Work out the finished part from the listing and answer in its coordinate system (mm). Face numbers are marked on the shaded views. A direction names the side the tool comes from. Give positions to 0.01 mm unless a question says otherwise; leave off trailing zeros. Loops run counter-clockwise (first coordinate to the right, second up) from the corner with the lowest first, then second, coordinate; pieces in that order, holes last. Notation, with made-up numbers: M 37,39.5 L 77,39.5 A20 cw 77,61.5 Z; hole C -27.5,22.25 d10. An arc over 180 degrees is marked long. Write item = value, one per line. Start each with the question number.
1. Flat-ended cylindrical pins translate along their axes: pin 1 Ø1.5 at (y, z) = (-14, 14) entering from -X; pin 2 Ø1 at (x, y) = (-30, -9) entering from +Z; pin 3 Ø0.5 at (y, z) = (20, -1.5) entering from -X; pin 4 Ø25 at (x, y) = (0, 0) entering from +Z. Find the tip coordinate at first contact, or state that the pin passes through.
2. The mould has two halves that part along X. Classify the marked faces 5, 6, 7 and 8: released by +X, released by -X, zero draft, split by the parting line, or undercut.
3. For the marked faces 1, 2, 3 and 4, determine the directions among +Z, -Z, +X, -X, +Y, -Y from which every point of the face is accessible in a straight line to the end or side of a thin tool.
4. Section B-B on x = 0 is taken. Determine the outline of the cut face in (y, z).
5. Section A-A on z = 13.25 is taken. Determine the outline of the cut face in (x, y).
6. Section C-C on y = 13 is taken. Determine the outline of the cut face in (x, z), plus the area to 3 significant figures.
7. Consider L1, parallel to X at y = -7, z = 5.5; L2, parallel to Y at x = 56, z = 21.85; L3, parallel to Z at x = 11.5, y = 19. Determine where each line is inside the solid, lowest interval first. Write a range as [from, to].
8. Section D-D on y = 0 is taken. Give the number of separate pieces and of enclosed holes in the cut face, plus the area to 3 significant figures.
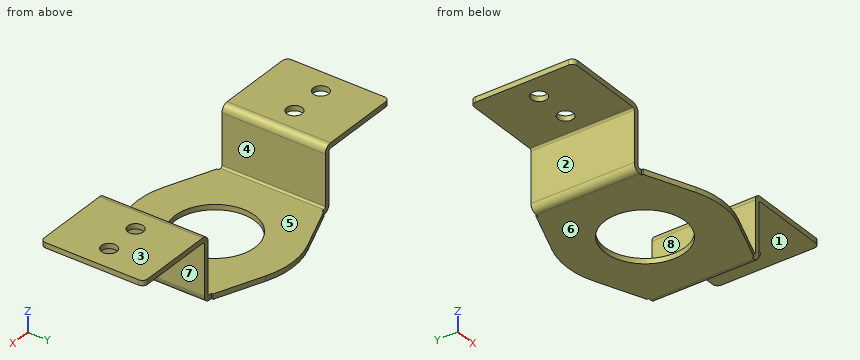
```python
from build123d import *

# Parameters (mm, degrees)
SKETCH1_R                       = 15.5
BASE_FLANGE1_DEPTH              = 2
EDGE_FLANGE1_STRIP_W            = 9.4732
EDGE_FLANGE1_STRIP_H            = 2
EDGE_FLANGE1_STRIP_CUT_DEPTH    = 40
EDGE_FLANGE1_RELIEF_W           = 10.4732
EDGE_FLANGE1_RELIEF_H           = 1
EDGE_FLANGE1_RELIEF_CUT_DEPTH   = 2
EDGE_FLANGE1_STRIP_2_W          = 9.4732
EDGE_FLANGE1_STRIP_2_H          = 2
EDGE_FLANGE1_STRIP_CUT_2_DEPTH  = 40
EDGE_FLANGE1_RELIEF_2_W         = 10.4732
EDGE_FLANGE1_RELIEF_2_H         = 1
EDGE_FLANGE1_RELIEF_CUT_2_DEPTH = 2
EDGE_FLANGE1_DEPTH              = 40
EDGE_FLANGE1_BEND_DEPTH         = 40
EDGE_FLANGE2_STRIP_W            = 9.4732
EDGE_FLANGE2_STRIP_H            = 2
EDGE_FLANGE2_STRIP_CUT_DEPTH    = 40
EDGE_FLANGE2_STRIP_2_W          = 9.4732
EDGE_FLANGE2_STRIP_2_H          = 2
EDGE_FLANGE2_STRIP_CUT_2_DEPTH  = 40
EDGE_FLANGE2_DEPTH              = 40
EDGE_FLANGE2_BEND_DEPTH         = 40
SKETCH17_R                      = 3
CUT_EXTRUDE1_DEPTH              = 10
FILLET1_R                       = 2


# Sheet-metal steps are written as plain solids
with BuildPart() as part:
    # Sketch1 → Base-Flange1 (new body)
    with BuildSketch(Plane.XY):
        with BuildLine():
            Line((-31, 20), (-11.034132012, 27.897095382))
            ThreePointArc((-11.034132012, 27.897095382), (0, 30), (11.034132012, 27.897095382))
            Line((11.034132012, 27.897095382), (31, 20))
            Line((31, 20), (31, -20))
            Line((31, -20), (11.034132012, -27.897095382))
            ThreePointArc((11.034132012, -27.897095382), (0, -30), (-11.034132012, -27.897095382))
            Line((-11.034132012, -27.897095382), (-31, -20))
            Line((-31, -20), (-31, 20))
        make_face()
        Circle(SKETCH1_R, mode=Mode.SUBTRACT)
    extrude(amount=-BASE_FLANGE1_DEPTH)

    # Edge-Flange1 strip (across the edge) → Edge-Flange1 strip cut (cut)
    with BuildSketch(Plane(origin=(-31, 20, 0), x_dir=(1, 0, 0), z_dir=(0, -1, 0))):
        with Locations((-4, -1)):
            Rectangle(EDGE_FLANGE1_STRIP_W, EDGE_FLANGE1_STRIP_H)
    extrude(amount=EDGE_FLANGE1_STRIP_CUT_DEPTH, mode=Mode.SUBTRACT)

    # Edge-Flange1 relief (on the sheet) → Edge-Flange1 relief cut (cut)
    with BuildSketch(Plane(origin=(-30.2634, 20, 0), x_dir=(1, 0, 0), z_dir=(0, 0, 1))):
        with Locations((-4.2366, 0.5)):
            Rectangle(EDGE_FLANGE1_RELIEF_W, EDGE_FLANGE1_RELIEF_H)
        with Locations((-4.2366, -40.5)):
            Rectangle(EDGE_FLANGE1_RELIEF_W, EDGE_FLANGE1_RELIEF_H)
    extrude(amount=-EDGE_FLANGE1_RELIEF_CUT_DEPTH, mode=Mode.SUBTRACT)

    # Edge-Flange1 strip 2 (across the edge) → Edge-Flange1 strip cut 2 (cut)
    with BuildSketch(Plane(origin=(31, -20, 0), x_dir=(-1, 0, 0), z_dir=(0, 1, 0))):
        with Locations((-4, -1)):
            Rectangle(EDGE_FLANGE1_STRIP_2_W, EDGE_FLANGE1_STRIP_2_H)
    extrude(amount=EDGE_FLANGE1_STRIP_CUT_2_DEPTH, mode=Mode.SUBTRACT)

    # Edge-Flange1 relief 2 (on the sheet) → Edge-Flange1 relief cut 2 (cut)
    with BuildSketch(Plane(origin=(30.2634, -20, 0), x_dir=(-1, 0, 0), z_dir=(0, 0, 1))):
        with Locations((-4.2366, 0.5)):
            Rectangle(EDGE_FLANGE1_RELIEF_2_W, EDGE_FLANGE1_RELIEF_2_H)
        with Locations((-4.2366, -40.5)):
            Rectangle(EDGE_FLANGE1_RELIEF_2_W, EDGE_FLANGE1_RELIEF_2_H)
    extrude(amount=-EDGE_FLANGE1_RELIEF_CUT_2_DEPTH, mode=Mode.SUBTRACT)

    # Edge-Flange1 section (across the edge) → Edge-Flange1 (add)
    with BuildSketch(Plane(origin=(-31, 20, 0), x_dir=(1, 0, 0), z_dir=(0, -1, 0))):
        with BuildLine():
            Line((-2, 0.7366), (-2, 21))
            Line((-2, 21), (0, 21))
            Line((0, 21), (0, 0.7366))
            ThreePointArc((0, 0.7366), (0.215745145, 0.215745145), (0.7366, 0))
            Line((0.7366, 0), (0.7366, -2))
            ThreePointArc((0.7366, -2), (-1.198468417, -1.198468417), (-2, 0.7366))
        make_face()
    extrude(amount=EDGE_FLANGE1_DEPTH)

    # Edge-Flange1 section 2 (across the edge) → Edge-Flange1 bend (add)
    with BuildSketch(Plane(origin=(31, -20, 0), x_dir=(-1, 0, 0), z_dir=(0, 1, 0))):
        with BuildLine():
            Line((-2, 0.7366), (-2, 21))
            Line((-2, 21), (0, 21))
            Line((0, 21), (0, 0.7366))
            ThreePointArc((0, 0.7366), (0.215745145, 0.215745145), (0.7366, 0))
            Line((0.7366, 0), (0.7366, -2))
            ThreePointArc((0.7366, -2), (-1.198468417, -1.198468417), (-2, 0.7366))
        make_face()
    extrude(amount=EDGE_FLANGE1_BEND_DEPTH)

    # Edge-Flange2 strip (across the edge) → Edge-Flange2 strip cut (cut)
    with BuildSketch(Plane(origin=(-33, -20, 21), x_dir=(0, 0, -1), z_dir=(0, 1, 0))):
        with Locations((-4, -1)):
            Rectangle(EDGE_FLANGE2_STRIP_W, EDGE_FLANGE2_STRIP_H)
    extrude(amount=EDGE_FLANGE2_STRIP_CUT_DEPTH, mode=Mode.SUBTRACT)

    # Edge-Flange2 strip 2 (across the edge) → Edge-Flange2 strip cut 2 (cut)
    with BuildSketch(Plane(origin=(33, 20, 21), x_dir=(0, 0, -1), z_dir=(0, -1, 0))):
        with Locations((-4, -1)):
            Rectangle(EDGE_FLANGE2_STRIP_2_W, EDGE_FLANGE2_STRIP_2_H)
    extrude(amount=EDGE_FLANGE2_STRIP_CUT_2_DEPTH, mode=Mode.SUBTRACT)

    # Edge-Flange2 section (across the edge) → Edge-Flange2 (add)
    with BuildSketch(Plane(origin=(-33, -20, 21), x_dir=(0, 0, -1), z_dir=(0, 1, 0))):
        with BuildLine():
            Line((-2, 0.7366), (-2, 32))
            Line((-2, 32), (0, 32))
            Line((0, 32), (0, 0.7366))
            ThreePointArc((0, 0.7366), (0.215745145, 0.215745145), (0.7366, 0))
            Line((0.7366, 0), (0.7366, -2))
            ThreePointArc((0.7366, -2), (-1.198468417, -1.198468417), (-2, 0.7366))
        make_face()
    extrude(amount=EDGE_FLANGE2_DEPTH)

    # Edge-Flange2 section 2 (across the edge) → Edge-Flange2 bend (add)
    with BuildSketch(Plane(origin=(33, 20, 21), x_dir=(0, 0, -1), z_dir=(0, -1, 0))):
        with BuildLine():
            Line((-2, 0.7366), (-2, 32))
            Line((-2, 32), (0, 32))
            Line((0, 32), (0, 0.7366))
            ThreePointArc((0, 0.7366), (0.215745145, 0.215745145), (0.7366, 0))
            Line((0.7366, 0), (0.7366, -2))
            ThreePointArc((0.7366, -2), (-1.198468417, -1.198468417), (-2, 0.7366))
        make_face()
    extrude(amount=EDGE_FLANGE2_BEND_DEPTH)

    # Sketch17 → Cut-Extrude1 (cut)
    with BuildSketch(Plane(origin=(0, 0, 21), x_dir=(-1, 0, 0), z_dir=(0, 0, -1))):
        with Locations((56, 0)):
            Circle(SKETCH17_R)
        with Locations((42, 0)):
            Circle(SKETCH17_R)
        with Locations((-56, 0)):
            Circle(SKETCH17_R)
        with Locations((-42, 0)):
            Circle(SKETCH17_R)
    extrude(amount=-CUT_EXTRUDE1_DEPTH, mode=Mode.SUBTRACT)

    # Fillet1
    fillet1_edges = [part.edges().sort_by_distance(p)[0] for p in [
        (-65, -20, 22),
        (-65, 20, 22),
        (65, 20, 22),
        (65, -20, 22),
    ]]
    fillet(fillet1_edges, radius=FILLET1_R)


solid = part.part
```
Verdict:
q1.pin_1 = -33
q1.pin_2 = 0.04
q1.pin_3 = -32.15
q1.pin_4 = through
q2.face_5 = undercut
q2.face_6 = zero draft
q2.face_7 = released by +X
q2.face_8 = undercut
q3.face_1 = -Z, +X, +Y, -Y
q3.face_2 = -Z, -X, +Y, -Y
q3.face_3 = +Z, +X, -X, +Y, -Y
q3.face_4 = +Z, +Y, -Y
q4.outline = M -30,-2 L -15.5,-2 L -15.5,0 L -30,0 Z; M 15.5,-2 L 30,-2 L 30,0 L 15.5,0 Z
q5.outline = M -33,-20 L -31,-20 L -31,20 L -33,20 Z; M 31,-20 L 33,-20 L 33,20 L 31,20 Z
q6.outline = M -65,21 L -33.74,21 A0.74 cw -33,20.26 L -33,0.74 A2.74 ccw -30.26,-2 L -8.44,-2 L -8.44,0 L -30.26,0 A0.74 cw -31,0.74 L -31,20.26 A2.74 ccw -33.74,23 L -65,23 Z; M 8.44,-2 L 30.26,-2 A2.74 ccw 33,0.74 L 33,20.26 A0.74 cw 33.74,21 L 65,21 L 65,23 L 33.74,23 A2.74 ccw 31,20.26 L 31,0.74 A0.74 cw 30.26,0 L 8.44,0 Z
q6.area = 312 mm2
q7.L1 = [-33, -31], [31, 33]
q7.L2 = [-20, -3], [3, 20]
q7.L3 = [-2, 0]
q8.separate_pieces = 6
q8.enclosed_holes = 0
q8.area = 236 mm2
